Part print with two shaded views. Sizes in mm from the minimum x, y, z corner. A direction names the side the tool comes from. Give positions to 0.01 mm unless a question says otherwise; leave off trailing zeros. Loops run counter-clockwise (first coordinate to the right, second up) from the corner with the lowest first, then second, coordinate; pieces in that order, holes last. Notation, with made-up numbers: M 59.25,45 L 72.25,45 A14 ccw 72.25,72 Z; hole C 80.25,12 d8. An arc over 180 degrees is marked long. Answer as a JSON object with one key per item and string values. Group by question number.
1. Slice it at A-A (x = 100). List the corners of the cut face in (y, z), then the cut area to 3 significant figures.
2. Slice it at B-B (z = 100). List the corners of the cut face in (x, y), then the cut area to 3 significant figures.
3. Slice it at D-D (x = 120). List the corners of the cut face in (y, z) (1 decimal), then the cut area to 3 significant figures.
4. Slice it at C-C (z = 192). List the corners of the cut face in (x, y).
5. Drill centre lines: line 1 along X through (y, z) = (16.5, 100); line 2 along X through (y, z) = (8.75, 98.5) (1 decimal); line 3 along Y through (x, z) = (189, 144). Where is each one in solid material? Low to high. Write a range as [from, to].
6. 3-axis set-ups, long thin cutter, end or side, ignore diameter. For the marked faces 1 and 2: which of +Z, -Z, +X, -X, +Y, -Y reach the whole face in a straight line?
7. Mould opens along Z. For the marked faces 3, 4 and 5 say: released by +Z, released by -Z, zero draft, split by the parting line, or undercut.
8. Drop flat-ended pins along their axis: pin 1 Ø4 at (x, y) = (142, 25) entering from -Z; pin 2 Ø12 at (x, y) = (156, 18.5) entering from +Z; pin 3 Ø13 at (x, z) = (34.95, 34.95) entering from -Y. Give the stop position or say it passes through.
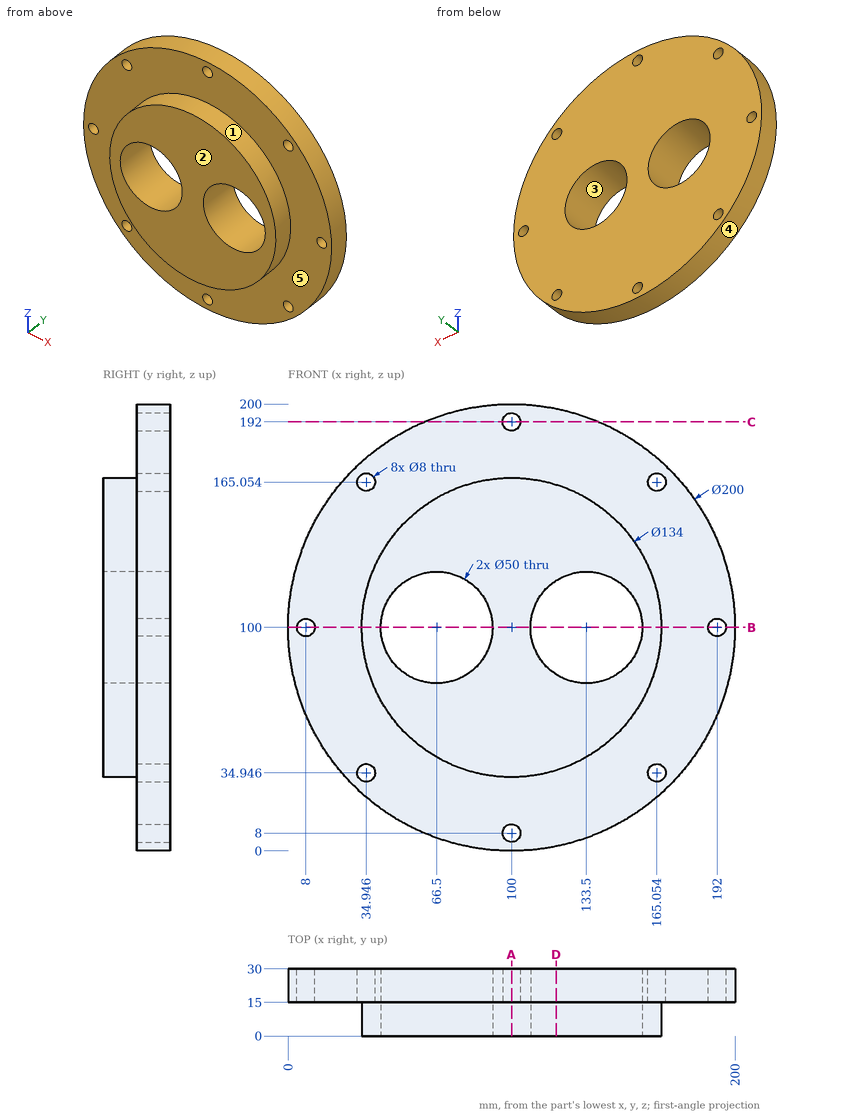
Established:
{
 "1": {"outline": "M 0,33 L 15,33 L 15,12 L 30,12 L 30,188 L 15,188 L 15,167 L 0,167 Z; M 15,0 L 30,0 L 30,4 L 15,4 Z; M 15,196 L 30,196 L 30,200 L 15,200 Z", "area": "4,770 mm^2"},
 "2": {"outline": "M 0,15 L 4,15 L 4,30 L 0,30 Z; M 12,15 L 33,15 L 33,0 L 41.5,0 L 41.5,30 L 12,30 Z; M 91.5,0 L 108.5,0 L 108.5,30 L 91.5,30 Z; M 158.5,0 L 167,0 L 167,15 L 188,15 L 188,30 L 158.5,30 Z; M 196,15 L 200,15 L 200,30 L 196,30 Z", "area": "1,770 mm^2"},
 "3": {"outline": "M 0,36.1 L 15,36.1 L 15,2 L 30,2 L 30,79 L 0,79 Z; M 0,121 L 30,121 L 30,198 L 15,198 L 15,163.9 L 0,163.9 Z", "area": "3,600 mm^2"},
 "4": {"outline": "M 60.81,15 L 96,15 L 96,30 L 60.81,30 Z; M 104,15 L 139.19,15 L 139.19,30 L 104,30 Z"},
 "5": {"line 1": "x = [0, 4], [12, 41.5], [91.5, 108.5], [158.5, 188], [196, 200]", "line 2": "x = [33, 41.5], [91.5, 108.5], [158.5, 167]", "line 3": "y = [15, 30]"},
 "6": {"face 1": "-Y", "face 2": "+Z, -Z, +X, -X, -Y"},
 "7": {"face 3": "undercut", "face 4": "split by the parting line", "face 5": "zero draft"},
 "8": {"pin 1": "stops at z = 8.35", "pin 2": "stops at z = 186.6", "pin 3": "stops at y = 15"}
}
